Source: CAD feature listing. Evaluate the final solid. Frame: model axes, mm. A direction names the side the tool comes from. Coordinates: 2 decimals unless noted, no trailing zeros. Order: outer loops, then holes, each group sorted by start corner. A loop starts at its lowest first (then second) coordinate and runs counter-clockwise, first axis right, second up.
Item 1: Mould query, pull axis X, two halves, no side actions, for faces 1 (the cylindrical face through (-13.986, 27.297, 2.535)), 2 (the cylindrical face through (0, -33, 2)), 3 (the flat face through (0, -0.5, 3)), 4 (the flat face through (4, 0, 0)). Classes: released by +X, released by -X, zero draft, split by the parting line, or undercut.
Item 2: Ray query, line 1 (Y direction, x = 2.5, z = 1.3); line 2 (X direction, y = 13.5, z = 0.6); line 3 (X direction, y = -20, z = 1.55). Return the intervals inside material, ascending.
Item 3: Contact query for flat-ended pins moving along their axis: P1, Ø2.5, axis at x = -1, z = 2, coming from the -Y side; P2, Ø2, axis at x = -16, z = 3.5, coming from the -Y side; P3, Ø1.5, axis at x = 1.5, z = 1.5, coming from the +Y side. Output: stop coordinate, or through.
Item 4: Section B-B on z = 1.4. State how many separate pieces and enclosed holes the cut face has, then the cut area to 3 significant figures.
Item 5: Reachability of faces 5 (the cylindrical face through (-16.91, -26.41, 2.54)), 6 (the flat face through (0, -15.5, 3)) from +Z, -Z, +X, -X, +Y, -Y: full face, straight path, thin tool, end or side. Return the list, or none.
Item 6: Section A-A on y = 1. Return the cut outline in (x, z).
Item 7: Section D-D on y = -23.5. Return the cut outline in (x, z).
Item 8: Section C-C on x = 14. Return the cut outline in (y, z), then the cut area to 3 significant figures.
from build123d import *

# Parameters (mm, degrees)
SKETCH1_R           = 33
BOSS_EXTRUDE1_DEPTH = 5
CUT_EXTRUDE3_START  = -10
CUT_EXTRUDE3_DEPTH  = 10
FILLET2_R           = 20
FILLET3_R           = 15
SKETCH11_W          = 7
SKETCH11_H          = 5
CUT_EXTRUDE4_DEPTH  = 10


with BuildPart() as part:
    # Sketch1 → Boss-Extrude1 (new body)
    with BuildSketch(Plane.XY):
        Circle(SKETCH1_R)
    extrude(amount=BOSS_EXTRUDE1_DEPTH)

    # Sketch10 → Cut-Extrude3 (cut)
    with BuildSketch(Plane.XY.offset(5).offset(CUT_EXTRUDE3_START)):
        with BuildLine():
            Line((-20, 26.248809497), (-20, -26.248809497))
            ThreePointArc((-20, -26.248809497), (-33, 0), (-20, 26.248809497))
        make_face()
        with BuildLine():
            Line((20, 26.248809497), (20, -26.248809497))
            ThreePointArc((20, -26.248809497), (33, 0), (20, 26.248809497))
        make_face()
    extrude(amount=CUT_EXTRUDE3_DEPTH, mode=Mode.SUBTRACT)

    # Fillet2
    fillet2_edges = [part.edges().sort_by_distance(p)[0] for p in [
        (-20, 26.248809497, 2.5),
        (20, 26.248809497, 2.5),
    ]]
    fillet(fillet2_edges, radius=FILLET2_R - 0.0001)  # a hair under: the kernel refuses the full size

    # Fillet3
    fillet3_edges = [part.edges().sort_by_distance(p)[0] for p in [
        (-20, -26.248809497, 2.5),
        (20, -26.248809497, 2.5),
    ]]
    fillet(fillet3_edges, radius=FILLET3_R)

    # Sketch11 → Cut-Extrude4 (cut)
    with BuildSketch(Plane.XY.offset(5)):
        with Locations((0, 2)):
            Rectangle(SKETCH11_W, SKETCH11_H)
        with Locations((0, -18)):
            Rectangle(SKETCH11_W, SKETCH11_H)
    extrude(amount=-CUT_EXTRUDE4_DEPTH, mode=Mode.SUBTRACT)


solid = part.part
Answer list:
1. face 1: released by -X
1. face 2: split by the parting line
1. face 3: undercut
1. face 4: zero draft
2. line 1: y = -32.91 to -20.5, -15.5 to -0.5, 4.5 to 32.84
2. line 2: x = -19.99 to 19.99
2. line 3: x = -19.75 to -3.5, 3.5 to 19.75
3. P1: stops at y = -33
3. P2: stops at y = -28.47
3. P3: stops at y = 32.99
4. separate pieces: 1
4. enclosed holes: 2
4. area: 2,280 mm2
5. face 5: +Z, -Z, -X, -Y
5. face 6: +Z, -Z
6. outline: (-20, 0) - (-3.5, 0) - (-3.5, 5) - (-20, 5) - close; (3.5, 0) - (20, 0) - (20, 5) - (3.5, 5) - close
7. outline: (-18.65, 0) - (18.65, 0) - (18.65, 5) - (-18.65, 5) - close
8. outline: (-29.29, 0) - (27.28, 0) - (27.28, 5) - (-29.29, 5) - close
8. area: 283 mm2
